Build history of the part. All positions in model axes, mm. A direction names the side the tool comes from. Round coordinates to 2 decimals unless told otherwise and drop trailing zeros. Write each loop counter-clockwise with the first axis right and the second up, starting at its lowest first coordinate (ties: lowest second). Pieces come first, ordered by that corner, then holes. Notation, with made-up numbers: (76.5, 55) - (93.5, 55) arc R32 ccw to (93.5, 83) - close; hole circle Ø4 at (60.5, 19.5). An arc over 180 degrees is marked (long way). One line per question, with ' | ' between items.
from build123d import *

# Parameters (mm, degrees)
F0_R      = 1.6
F1_DEPTH  = 2.45
F4_DEPTH  = 8
F6_R      = 1.6
F7_DEPTH  = 25
F8_DEPTH  = 11
F9_W      = 7.5
F9_H      = 2.5
F10_DEPTH = 14.29


with BuildPart() as f1:
    # F0 (on Top) → F1 (new body)
    with BuildSketch(Plane.XY):
        with BuildLine():
            Line((-6.325, -2.475), (13.825, -2.475))
            ThreePointArc((13.825, -2.475), (15.5397339444, -1.7647339444), (16.25, -0.05))
            Line((16.25, -0.05), (16.25, 0.05))
            ThreePointArc((16.25, 0.05), (15.5397339444, 1.7647339444), (13.825, 2.475))
            Line((13.825, 2.475), (-6.325, 2.475))
            Line((-6.325, 2.475), (-8.75, 2.475))
            Line((-8.75, 2.475), (-13.825, 2.475))
            Line((-13.825, 2.475), (-16.25, 2.475))
            Line((-16.25, 2.475), (-16.25, -2.475))
            Line((-16.25, -2.475), (-13.825, -2.475))
            Line((-13.825, -2.475), (-6.325, -2.475))
        make_face()
        with Locations((13.55, 0)):
            Circle(F0_R, mode=Mode.SUBTRACT)
    extrude(amount=F1_DEPTH)

    # F2: F1 across plane


with BuildPart() as f1_1:
    add(f1.part)
    add(f1.part.mirror(Plane.XY))

    # F3 (on face) → F4 (join)
    with BuildSketch(Plane.XZ.offset(2.475)):
        with BuildLine():
            Line((-24.75, 0), (-16.25, 0))
            Line((-16.25, 0), (-16.25, 2.45))
            Line((-16.25, 2.45), (-16.25, 4))
            ThreePointArc((-16.25, 4), (-16.5428932188, 4.7071067812), (-17.25, 5))
            Line((-17.25, 5), (-23.75, 5))
            ThreePointArc((-23.75, 5), (-24.4571067812, 4.7071067812), (-24.75, 4))
            Line((-24.75, 4), (-24.75, 0))
        make_face()
    extrude(amount=-F4_DEPTH)

    # F5: F1 across plane


with BuildPart() as f1_2:
    add(f1_1.part)
    add(f1_1.part.mirror(Plane.XY))

    # F6 (on face) → F7 (cut)
    with BuildSketch(Plane.XZ.offset(2.475)):
        with Locations((-20.5, 0)):
            Circle(F6_R)
    extrude(amount=-F7_DEPTH, mode=Mode.SUBTRACT)

    # F8 (add): a face of the model
    f8_faces = [f1_2.faces().sort_by_distance(p)[0] for p in [
        (-24.3643032252, 5.525, 4.6143032252),
    ]]
    extrude(f8_faces, amount=-F8_DEPTH)

    # F9 (on face) → F10 (cut)
    with BuildSketch(Plane(origin=(0, 0, -5), x_dir=(1, 0, 0), z_dir=(0, 0, -1))):
        with Locations((-21.55, 1.25)):
            Rectangle(F9_W, F9_H)
        with Locations((-21.55, -1.25)):
            Rectangle(F9_W, F9_H)
    extrude(amount=-F10_DEPTH, mode=Mode.SUBTRACT)


solid = f1_2.part
Q1. Saw through at B-B, the plane x = -20.5. List the corners of the cut face in (y, z) (3 decimals).
Found:
outline: (-5.475, -5) - (-2.5, -5) - (-2.5, -1.6) - (-5.475, -1.6) - close; (-5.475, 1.6) - (-2.5, 1.6) - (-2.5, 5) - (-5.475, 5) - close; (2.5, -5) - (5.525, -5) - (5.525, -1.6) - (2.5, -1.6) - close; (2.5, 1.6) - (5.525, 1.6) - (5.525, 5) - (2.5, 5) - close
Q2. Saw through at D-D, the plane z = -3.25. List the corners of the cut face in (x, y) (3 decimals), then the cut area to 4 significant figures.
Found:
outline: (-24.75, -5.475) - (-16.25, -5.475) - (-16.25, 5.525) - (-24.75, 5.525) - (-24.75, 2.5) - (-17.8, 2.5) - (-17.8, -2.5) - (-24.75, -2.5) - close | area: 58.75 mm^2
Q3. Pull direction X, two halves, no side cores. Call faces 6 (the cylindrical face through (15.6, 1.7, 0)), 7 (the cylindrical face through (-21.68, -3.97, 1.08)), 8 (the cylindrical face through (-24.449, 4.034, -4.715)), 9 (the flat face through (-22, 2.5, 1)): +X half, -X half, draft (parallel to the pull), parting line (faces both ways), or undercut.
Found:
face 6: +X half | face 7: undercut | face 8: -X half | face 9: draft
Q4. Drill centre lines: L1, parallel to Y at x = 13.55, z = -1.3 (3 decimals); L2, parallel to Z at x = -20.5, y = -3.75; L3, parallel to X at y = -4.8, z = 0. Where is each one in solid material? Low to high. Write a range as from..to.
Found:
L1: -2.475..-1.6, 1.6..2.475 | L2: -5..-1.6, 1.6..5 | L3: -24.75..-22.1, -18.9..-16.25
Q5. Saw through at A-A, the plane z = 0. List the corners of the cut face in (x, y) (3 decimals), then the cut area to 3 significant figures.
Found:
outline: (-24.75, -5.475) - (-22.1, -5.475) - (-22.1, -2.5) - (-24.75, -2.5) - close; (-24.75, 2.5) - (-22.1, 2.5) - (-22.1, 5.525) - (-24.75, 5.525) - close; (-18.9, -5.475) - (-16.25, -5.475) - (-16.25, -2.475) - (13.825, -2.475) arc R2.425 ccw to (16.25, -0.05) - (16.25, 0.05) arc R2.425 ccw to (13.825, 2.475) - (-16.25, 2.475) - (-16.25, 5.525) - (-18.9, 5.525) - (-18.9, 2.5) - (-17.8, 2.5) - (-17.8, -2.5) - (-18.9, -2.5) - close; hole circle Ø3.2 at (13.55, 0) | area: 190 mm^2
Q6. Drop flat-ended pins along their axis: pin 1 (4 mm diameter, centred on x = 7, y = 0, fed in from +Z); pin 2 (4 mm diameter, centred on y = 0, z = 0, fed in from -X); pin 3 (4 mm diameter, centred on x = -1.5, y = 0, fed in from -Z). Give the stop position or say it passes through.
Found:
pin 1: z = 2.45 | pin 2: x = -17.8 | pin 3: z = -2.45
Q7. Which spindle directions (+Z, -Z, +X, -X, +Y, -Y) get a long thin tool onto all of the face, cutting with end or side? Do faces 1 (the cylindrical face through (-24.449, -3.967, 4.715)), 2 (the flat face through (-17.8, 0, 0)), 3 (the flat face through (-16.25, 3, 0)), 4 (the flat face through (-1, -2.475, 0)), 5 (the cylindrical face through (-21.68, 4.03, 1.08)). Say none if no direction does.
Found:
face 1: +Z, -X, +Y, -Y | face 2: +Z, -Z, -X | face 3: +X | face 4: +Z, -Z, +X, -Y | face 5: +Y, -Y
Q8. Saw through at C-C, the plane y = -4.5. List the corners of the cut face in (x, z), then the cut area to 3 significant figures.
Found:
outline: (-24.75, -4) arc R1 ccw to (-23.75, -5) - (-17.25, -5) arc R1 ccw to (-16.25, -4) - (-16.25, 4) arc R1 ccw to (-17.25, 5) - (-23.75, 5) arc R1 ccw to (-24.75, 4) - close; hole circle Ø3.2 at (-20.5, 0) | area: 76.1 mm^2
